```python
from build123d import *

# Parameters (mm, degrees)
BOSS_EXTRUDE1_DEPTH = 2.5
SKETCH2_R           = 1
CUT_EXTRUDE1_DEPTH  = 5
SKETCH3_R           = 1
CUT_EXTRUDE2_DEPTH  = 5
SKETCH5_R           = 1
BOSS_EXTRUDE2_DEPTH = 5
SKETCH6_W           = 2.5
SKETCH6_H           = 2.5
BOSS_EXTRUDE3_DEPTH = 25
SKETCH7_R           = 1
CUT_EXTRUDE3_DEPTH  = 5


with BuildPart() as part:
    # Sketch1 → Boss-Extrude1 (new body)
    with BuildSketch(Plane.XY):
        Polygon((-5, 0), (0, 0), (3.830222216, 3.213938048), (5.465982834, 1.323359513), (0.909480399, -2.5), (-5, -2.5), align=None)
    extrude(amount=BOSS_EXTRUDE1_DEPTH)

    # Sketch2 → Cut-Extrude1 (cut)
    with BuildSketch(Plane(origin=(3.780724263, 3.271146765, 0), x_dir=(0, 0, -1), z_dir=(0.7562314141303861, 0.6543042474891606, 0))):
        with Locations(Location((-1.25, -1.325649749, 0), (0, 0, 90))):
            Circle(SKETCH2_R)
    extrude(amount=-CUT_EXTRUDE1_DEPTH, mode=Mode.SUBTRACT)

    # Sketch3 → Cut-Extrude2 (cut)
    with BuildSketch(Plane.ZY.offset(5)):
        with Locations((1.25, -1.25)):
            Circle(SKETCH3_R)
    extrude(amount=-CUT_EXTRUDE2_DEPTH, mode=Mode.SUBTRACT)

    # Sketch5 → Boss-Extrude2 (add)
    with BuildSketch(Plane.ZY.offset(5)):
        with Locations((1.25, -1.25)):
            Circle(SKETCH5_R)
    extrude(amount=-BOSS_EXTRUDE2_DEPTH)

    # Sketch6 → Boss-Extrude3 (add)
    with BuildSketch(Plane.ZY.offset(5)):
        with Locations((1.25, -1.25)):
            Rectangle(SKETCH6_W, SKETCH6_H)
    extrude(amount=BOSS_EXTRUDE3_DEPTH)

    # Sketch7 → Cut-Extrude3 (cut)
    with BuildSketch(Plane.ZY.offset(30)):
        with Locations((1.25, -1.25)):
            Circle(SKETCH7_R)
    extrude(amount=-CUT_EXTRUDE3_DEPTH, mode=Mode.SUBTRACT)


solid = part.part
```
Input: part model. Units: mm. Frame: model coordinates. A direction names the side the tool comes from. Round coordinates to 2 decimals unless told otherwise and drop trailing zeros. Write each loop counter-clockwise with the first axis right and the second up, starting at its lowest first coordinate (ties: lowest second). Pieces come first, ordered by that corner, then holes. Notation, with made-up numbers: (77, 76.5) - (135, 76.5) arc R17 cw to (135, 95.5) - close; hole circle Ø11 at (-21.75, 17). An arc over 180 degrees is marked (long way). Write item = value, one per line.
(1) Section query C-C on x = -8.5. Output: boundary loops of the cut face in (y, z), then the cut area to 3 significant figures.
Geometry check:
outline = (-2.5, 0) - (0, 0) - (0, 2.5) - (-2.5, 2.5) - close
area = 6.25 mm^2
(2) Section query B-B on z = 1.25. Output: boundary loops of the cut face in (x, y), then the cut area to 3 significant figures.
Geometry check:
outline = (-30, -2.5) - (0.91, -2.5) - (5.47, 1.32) - (5.3, 1.51) - (1.52, -1.76) - (0.21, -0.25) - (3.99, 3.02) - (3.83, 3.21) - (0, 0) - (-30, 0) - (-30, -0.25) - (-25, -0.25) - (-25, -2.25) - (-30, -2.25) - close
area = 69.8 mm^2
(3) Section query A-A on x = -26.5. Output: boundary loops of the cut face in (y, z).
Geometry check:
outline = (-2.5, 0) - (0, 0) - (0, 2.5) - (-2.5, 2.5) - close; hole circle Ø2 at (-1.25, 1.25)
(4) Contact query for flat-ended pins moving along their axis: pin 1 Ø1.2 at (x, z) = (-17, 2) entering from +Y; pin 2 Ø0.6 at (y, z) = (-1, 1.5) entering from -X; pin 3 Ø1 at (y, z) = (-1, 0.5) entering from -X. Output: stop coordinate, or through.
Geometry check:
pin_1 = 0
pin_2 = -25
pin_3 = -30
(5) Access query for faces 5 (the flat face through (-14, -2.5, 1)), 6 (the flat face through (0.876, -1.013, 1.264)), 7 (the flat face through (-25, -1, 1)), 8 (the flat face through (-15, 0, 1)). Directions: +Z, -Z, +X, -X, +Y, -Y. A direction counts if a zero-diameter tool reaches every point of the face in a straight line with its end or side. Return the directions, or none.
Geometry check:
face_5 = +Z, -Z, +X, -X, -Y
face_6 = none
face_7 = -X
face_8 = +Z, -Z, -X, +Y
(6) Material intervals for probe 1 along Z at (x, y) = (4.5, 2.05); probe 2 along Y at (x, z) = (-10, 1.7); probe 3 along X at (y, z) = (0.75, 2.05), sorted ascending.
Geometry check:
probe_1 = 0 to 0.25, 2.25 to 2.5
probe_2 = -2.5 to 0
probe_3 = 0.89 to 1.98, 3.81 to 4.78
(7) Pull-direction query (Z, two-part tool) for faces 1 (the cylindrical face through (-27.535, -2.226, 1.033)), 2 (the flat face through (-12, -1, 2.5)), 3 (the flat face through (3.22, -0.56, 1.23)), 4 (the flat face through (-12, -1, 0)); classes: +Z half, -Z half, draft (parallel to the pull), parting line (faces both ways), or undercut.
Geometry check:
face_1 = undercut
face_2 = +Z half
face_3 = draft
face_4 = -Z half
